```python
from build123d import *

# Parameters (mm, degrees)
BOSS_EXTRUDE1_DEPTH                           = 80
SKETCH2_W                                     = 40
SKETCH2_H                                     = 40
CUT_EXTRUDE1_DEPTH                            = 60
SKETCH3_R                                     = 9.75
CUT_EXTRUDE2_DEPTH                            = 70
CBORE_FOR_M2_CHEESE_SLOTTED_HEAD3_D           = 2.4
CBORE_FOR_M2_CHEESE_SLOTTED_HEAD3_CBORE_D     = 4.8
CBORE_FOR_M2_CHEESE_SLOTTED_HEAD3_CBORE_DEPTH = 1.4


with BuildPart() as part:
    # Sketch1 → Boss-Extrude1 (new body)
    with BuildSketch(Plane(origin=(0, 0, 0), x_dir=(0, 0, -1), z_dir=(1, 0, 0))):
        with BuildLine():
            Line((0, 0), (150, 0))
            ThreePointArc((150, 0), (166, 16), (150, 32))
            Line((150, 32), (0, 32))
            Line((0, 32), (0, 0))
        make_face()
    extrude(amount=BOSS_EXTRUDE1_DEPTH)

    # Sketch2 → Cut-Extrude1 (cut)
    with BuildSketch(Plane(origin=(0, 32, 0), x_dir=(1, 0, 0), z_dir=(0, 1, 0))):
        with Locations((40, 150)):
            Rectangle(SKETCH2_W, SKETCH2_H)
    extrude(amount=-CUT_EXTRUDE1_DEPTH, mode=Mode.SUBTRACT)

    # Sketch3 → Cut-Extrude2 (cut)
    with BuildSketch(Plane(origin=(80, 0, 0), x_dir=(0, 0, -1), z_dir=(1, 0, 0))):
        with Locations((150, 16)):
            Circle(SKETCH3_R)
    extrude(amount=-CUT_EXTRUDE2_DEPTH, mode=Mode.SUBTRACT)

    # CBORE for M2 Cheese Slotted Head3 (through all)
    with Locations(Plane(origin=(0, 24, -150), x_dir=(0, 0, -1), z_dir=(-1, 0, 0))):
        with Locations((0, 0), (-5.656854249, 2.343145751), (-8, 8), (-5.656854249, 13.656854249), (0, 16), (5.656854249, 13.656854249), (8, 8), (5.656854249, 2.343145751)):
            CounterBoreHole(CBORE_FOR_M2_CHEESE_SLOTTED_HEAD3_D / 2, CBORE_FOR_M2_CHEESE_SLOTTED_HEAD3_CBORE_D / 2, CBORE_FOR_M2_CHEESE_SLOTTED_HEAD3_CBORE_DEPTH)


solid = part.part
```
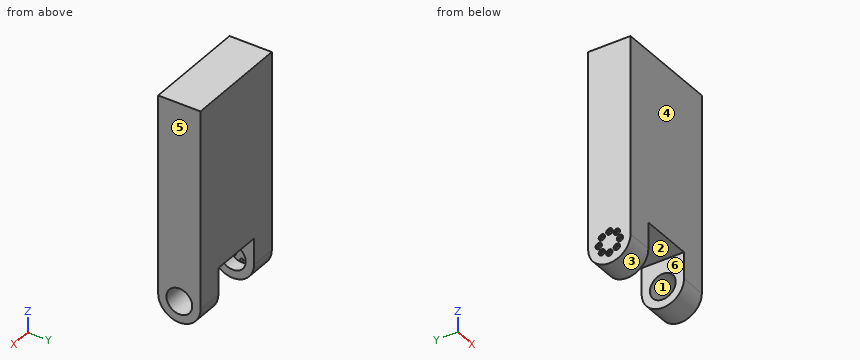
Work out the finished part from the listing and answer in its coordinate system (mm). Face numbers are marked on the shaded views. A direction names the side the tool comes from. Give positions to 0.01 mm unless a question says otherwise; leave off trailing zeros. Write each loop counter-clockwise with the first axis right and the second up, starting at its lowest first coordinate (ties: lowest second). Pieces come first, ordered by that corner, then holes. Notation, with made-up numbers: (-29.75, 72.25) -> (-6.75, 72.25) arc R8 ccw to (-6.75, 82.25) -> close; hole circle Ø5 at (51.25, 18.5). An arc over 180 degrees is marked (long way). Write item = value, one per line.
Q1. Consider line 1 along Y through (x, z) = (3.5, -150); line 2 along Z through (x, y) = (3.5, 16); line 3 along Y through (x, z) = (73.5, -150). Determine where each line is inside the solid, lowest interval first.
Computed values:
line_1 = 0 to 6.8, 9.2 to 22.8, 25.2 to 32
line_2 = -166 to -159.2, -156.8 to -143.2, -140.8 to 0
line_3 = 0 to 6.25, 25.75 to 32
Q2. Section C-C on x = 50 is taken. Determine the outline of the cut face in (y, z), and give its area (3 significant figures).
Computed values:
outline = (0, -130) -> (32, -130) -> (32, 0) -> (0, 0) -> close
area = 4,160 mm^2
Q3. A tool of negligible diameter and unlimited length cuts with its end or side. For the marked faces 1, 2 and 3, from which of +Z, -Z, +X, -X, +Y, -Y can it reach the whole face along a straight path? Write none if from no direction.
Computed values:
face_1 = +X
face_2 = -Z, +Y, -Y
face_3 = -Z, +X, -X
Q4. For a pull along X with two mould halves and no side action, classify the marked faces 4, 5 and 6 as pulls with the +X half, pulls with the -X half, needs draft (parallel to the pull), parting line crosses it, or undercut.
Computed values:
face_4 = needs draft
face_5 = pulls with the +X half
face_6 = undercut
Q5. Flat-ended cylindrical pins translate along their axes: pin 1 Ø3 at (y, z) = (8, -150) entering from -X; pin 2 Ø2 at (y, z) = (21.66, -155.66) entering from +X; pin 3 Ø3 at (y, z) = (10.34, -144.34) entering from +X; pin 4 Ø5 at (x, y) = (10, 22) entering from -Z. Find the tip coordinate at first contact, or state that the pin passes through.
Computed values:
pin_1 = 1.4
pin_2 = through
pin_3 = 10
pin_4 = -165.61
Q6. Section A-A on x = 65.5 is taken. Determine the outline of the cut face in (y, z), and give its area (3 significant figures).
Computed values:
outline = (0, -150) arc R16 ccw to (32, -150) -> (32, 0) -> (0, 0) -> close; hole circle Ø19.5 at (16, -150)
area = 4,900 mm^2
Q7. Section B-B on y = 3.5 is taken. Determine the outline of the cut face in (x, z).
Computed values:
outline = (0, -159.99) -> (20, -159.99) -> (20, -130) -> (60, -130) -> (60, -159.99) -> (80, -159.99) -> (80, 0) -> (0, 0) -> close
